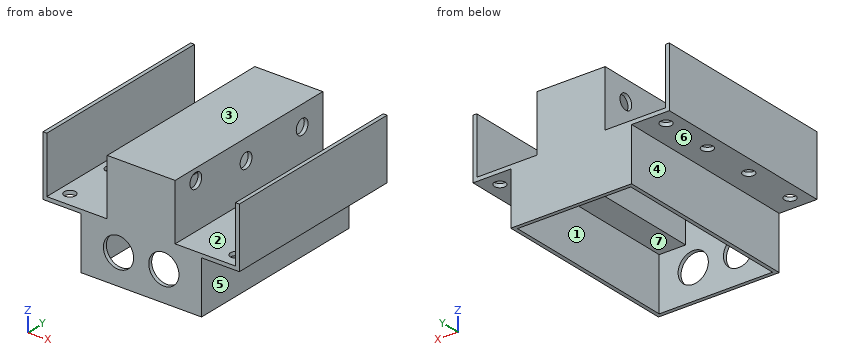
```python
from build123d import *

# Parameters (mm, degrees)
ESQUISSE1_W             = 90
ESQUISSE1_H             = 250
BOSS_EXTRU_1_DEPTH      = 5
ESQUISSE2_W             = 90
ESQUISSE2_H             = 250
ESQUISSE2_W_2           = 80
ESQUISSE2_H_2           = 240
BOSS_EXTRU_2_DEPTH      = 70
BOSS_EXTRU_3_DEPTH      = 5
ESQUISSE4_R             = 10
ENL_V_MAT_EXTRU_2_DEPTH = 171
ESQUISSE5_W             = 80
ESQUISSE5_H             = 250
BOSS_EXTRU_4_DEPTH      = 5
ESQUISSE6_W             = 80
ESQUISSE6_H             = 250
BOSS_EXTRU_5_DEPTH      = 5
ESQUISSE7_W             = 160
ESQUISSE7_H             = 250
ESQUISSE7_W_2           = 150
ESQUISSE7_H_2           = 240
BOSS_EXTRU_6_DEPTH      = 70
ESQUISSE10_R            = 7.5
ENL_V_MAT_EXTRU_3_DEPTH = 50
ESQUISSE12_R            = 20
ENL_V_MAT_EXTRU_4_DEPTH = 10


with BuildPart() as part:
    # Esquisse1 → Boss.-Extru.1 (new body)
    with BuildSketch(Plane.XY):
        with Locations((-45, 125)):
            Rectangle(ESQUISSE1_W, ESQUISSE1_H)
    extrude(amount=BOSS_EXTRU_1_DEPTH)

    # Esquisse2 → Boss.-Extru.2 (add)
    with BuildSketch(Plane(origin=(0, 0, 0), x_dir=(-1, 0, 0), z_dir=(0, 0, -1))):
        with Locations((45, 125)):
            Rectangle(ESQUISSE2_W, ESQUISSE2_H)
        with Locations((45, 125)):
            Rectangle(ESQUISSE2_W_2, ESQUISSE2_H_2, mode=Mode.SUBTRACT)
    extrude(amount=BOSS_EXTRU_2_DEPTH)

    # Esquisse3 → Boss.-Extru.3 (add)
    with BuildSketch(Plane(origin=(0, 0, -70), x_dir=(-1, 0, 0), z_dir=(0, 0, -1))):
        Polygon((6.025463364, 250), (-80, 250), (-80, 0), (-15, 0), (45, 0), (45, 5), (5, 5), (5, 245), (45, 245), (45, 250), align=None)
    boss_extru_3 = extrude(amount=BOSS_EXTRU_3_DEPTH)

    # Symétrie1: Boss.-Extru.3 across plane
    add(boss_extru_3.mirror(Plane(origin=(-45, 245, -75), x_dir=(0, 0, 1), z_dir=(1, 0, 0))))

    # Esquisse4 → Enlèv. mat.-Extru.2 (cut, through all)
    with BuildSketch(Plane.ZY.offset(90)):
        with Locations((-22, 215)):
            Circle(ESQUISSE4_R)
        with Locations((-22, 120)):
            Circle(ESQUISSE4_R)
        with Locations((-10, 35)):
            Circle(ESQUISSE4_R)
    extrude(amount=-ENL_V_MAT_EXTRU_2_DEPTH, mode=Mode.SUBTRACT)

    # Esquisse5 → Boss.-Extru.4 (add)
    with BuildSketch(Plane(origin=(80, 0, 0), x_dir=(0, 0, -1), z_dir=(1, 0, 0))):
        with Locations((35, 125)):
            Rectangle(ESQUISSE5_W, ESQUISSE5_H)
    extrude(amount=BOSS_EXTRU_4_DEPTH)

    # Esquisse6 → Boss.-Extru.5 (add)
    with BuildSketch(Plane.ZY.offset(170)):
        with Locations((-35, 125)):
            Rectangle(ESQUISSE6_W, ESQUISSE6_H)
    extrude(amount=BOSS_EXTRU_5_DEPTH)

    # Esquisse7 → Boss.-Extru.6 (add)
    with BuildSketch(Plane(origin=(0, 0, -75), x_dir=(-1, 0, 0), z_dir=(0, 0, -1))):
        with Locations((45, 125)):
            Rectangle(ESQUISSE7_W, ESQUISSE7_H)
        with Locations((45, 125)):
            Rectangle(ESQUISSE7_W_2, ESQUISSE7_H_2, mode=Mode.SUBTRACT)
    extrude(amount=BOSS_EXTRU_6_DEPTH)

    # Esquisse10 → Enlèv. mat.-Extru.3 (cut)
    with BuildSketch(Plane(origin=(0, 0, -75), x_dir=(-1, 0, 0), z_dir=(0, 0, -1))):
        with Locations((155, 230)):
            Circle(ESQUISSE10_R)
        with Locations((-65, 230)):
            Circle(ESQUISSE10_R)
        with Locations((-65, 160)):
            Circle(ESQUISSE10_R)
        with Locations((155, 160)):
            Circle(ESQUISSE10_R)
        with Locations((-65, 90)):
            Circle(ESQUISSE10_R)
        with Locations((155, 90)):
            Circle(ESQUISSE10_R)
        with Locations((-65, 20)):
            Circle(ESQUISSE10_R)
        with Locations((155, 20)):
            Circle(ESQUISSE10_R)
    extrude(amount=-ENL_V_MAT_EXTRU_3_DEPTH, mode=Mode.SUBTRACT)

    # Esquisse12 → Enlèv. mat.-Extru.4 (cut)
    with BuildSketch(Plane.XZ):
        with Locations((-15, -104.868866133)):
            Circle(ESQUISSE12_R)
        with Locations((-75, -104.868866133)):
            Circle(ESQUISSE12_R)
    extrude(amount=-ENL_V_MAT_EXTRU_4_DEPTH, mode=Mode.SUBTRACT)


solid = part.part
```
Part model, mm, in its own coordinate system. Face numbers are marked on the shaded views. A direction names the side the tool comes from. Give positions to 0.01 mm unless a question says otherwise; leave off trailing zeros. Write each loop counter-clockwise with the first axis right and the second up, starting at its lowest first coordinate (ties: lowest second). Pieces come first, ordered by that corner, then holes. Notation, with made-up numbers: M -1.75,88.25 L 14.25,88.25 A19 ccw 14.25,94.25 Z; hole C 46.5,63.25 d8. An arc over 180 degrees is marked long. Use CSV: the item, a comma, the result in double quotes.
Item 1: Slice it at C-C on x = -15. Write the cut outline in (y, z), plus the area to 3 significant figures.
Taken from the geometry:
outline,"M 0,-145 L 5,-145 L 5,-124.87 L 0,-124.87 Z; M 0,-84.87 L 5,-84.87 L 5,0 L 245,0 L 245,-145 L 250,-145 L 250,5 L 0,5 Z"
area,"2,500 mm²"
Item 2: Drill centre lines: probe 1 along X at (y, z) = (210, -1); probe 2 along Y at (x, z) = (-88, -22); probe 3 along Y at (x, z) = (-74.5, -55). Where is each one in solid material? Low to high.
Taken from the geometry:
probe 1,"x = -175 to -170, -90 to -85, -5 to 0, 80 to 85"
probe 2,"y = 0 to 110, 130 to 205, 225 to 250"
probe 3,"y = 0 to 5, 245 to 250"
Item 3: Which spindle directions (+Z, -Z, +X, -X, +Y, -Y) get a long thin tool onto all of the face, cutting with end or side? Do the marked faces 1, 2 and 3. Say none if no direction does.
Taken from the geometry:
face 1,"-Z"
face 2,"+Z, +Y, -Y"
face 3,"+Z, +X, -X, +Y, -Y"
Item 4: Pull direction X, two halves, no side cores. Call the marked faces 4, 5, 6 and 7: +X half, -X half, draft (parallel to the pull), parting line (faces both ways), or undercut.
Taken from the geometry:
face 4,"-X half"
face 5,"+X half"
face 6,"draft"
face 7,"undercut"
Item 5: Pin check, flat tips, straight feed: P1, Ø17, axis at x = -155, y = 20, coming from the -Z side; P2, Ø21, axis at y = 149.5, z = -123, coming from the +X side; P3, Ø13.5, axis at x = -155, y = 160, coming from the +Z side; P4, Ø6, axis at x = 34, y = 134.5, coming from the +Z side. Stop position of each tip, or through.
Taken from the geometry:
P1,"stops at z = -75"
P2,"stops at x = 35"
P3,"passes through"
P4,"stops at z = -70"
Item 6: Slice it at A-A on z = -52. Write the cut outline in (x, y), plus the area to 3 significant figures.
Taken from the geometry:
outline,"M -175,0 L -170,0 L -170,250 L -175,250 Z; M -90,0 L 0,0 L 0,250 L -90,250 Z; M 80,0 L 85,0 L 85,250 L 80,250 Z; hole M -85,5 L -5,5 L -5,245 L -85,245 Z"
area,"5,800 mm²"
Item 7: Slice it at B-B on y = 120. State how many separate pieces and enclosed holes the cut face has, plus the area to 3 significant figures.
Taken from the geometry:
separate pieces,"3"
enclosed holes,"0"
area,"3,300 mm²"
Item 8: Slice it at D-D on x = -155. Write the cut outline in (y, z).
Taken from the geometry:
outline,"M 0,-75 L 12.5,-75 L 12.5,-70 L 0,-70 Z; M 27.5,-75 L 82.5,-75 L 82.5,-70 L 27.5,-70 Z; M 97.5,-75 L 152.5,-75 L 152.5,-70 L 97.5,-70 Z; M 167.5,-75 L 222.5,-75 L 222.5,-70 L 167.5,-70 Z; M 237.5,-75 L 250,-75 L 250,-70 L 237.5,-70 Z"
